Source: CAD feature listing. Evaluate the final solid. Frame: model axes, mm. A direction names the side the tool comes from. Round coordinates to 2 decimals unless told otherwise and drop trailing zeros. Write each loop counter-clockwise with the first axis right and the second up, starting at its lowest first coordinate (ties: lowest second). Pieces come first, ordered by that corner, then holes. Notation, with made-up numbers: (-31, 72.25) - (4, 72.25) arc R5 ccw to (4, 81.25) - close; hole circle Ø3 at (21, 54.25). An arc over 180 degrees is marked (long way). Write item = value, one per line. Start each with the question number.
```python
from build123d import *

# Parameters (mm, degrees)
SKETCH_1_R      = 2.5
SKETCH_1_R_2    = 2.25
EXTRUDE_1_DEPTH = 2.5
FILLET_1_R      = 2


with BuildPart() as part:
    # 草图1 → 拉伸1 (new body)
    with BuildSketch(Plane.XY):
        with BuildLine():
            Line((-3.85, -23), (-3.85, -7.578093428))
            ThreePointArc((-3.85, -7.578093428), (0.055897166, 8.499816204), (3.75, -7.628073151))
            Line((3.75, -7.628073151), (3.75, -23))
            Line((3.75, -23), (-3.85, -23))
        make_face()
        Circle(SKETCH_1_R, mode=Mode.SUBTRACT)
        with Locations((0, -19)):
            Circle(SKETCH_1_R_2, mode=Mode.SUBTRACT)
    extrude(amount=EXTRUDE_1_DEPTH)

    # 圆角1
    fillet_1_edges = [part.edges().sort_by_distance(p)[0] for p in [
        (-3.85, -23, 1.25),
        (-3.85, -7.578093428, 1.25),
        (3.75, -7.628073151, 1.25),
        (3.75, -23, 1.25),
    ]]
    fillet(fillet_1_edges, radius=FILLET_1_R)


solid = part.part
```
(1) Section A-A (y = 0). Return the cut outline in (x, z).
(2) Reachability of faces 1 (the flat face through (-3.85, -15, 1)), 2 (the flat face through (3.75, -15, 1)), 3 (the cylindrical face through (-0.488, -21.196, 1.232)) from +Z, -Z, +X, -X, +Y, -Y: full face, straight path, thin tool, end or side. Return the list, or none.
(3) Section D-D (y = -19). Return the cut outline in (x, z).
(4) Contact query for flat-ended pins moving along their axis: P1, Ø1, axis at y = 1.5, z = 1, coming from the -X side; P2, Ø0.8, axis at y = -15, z = 1.5, coming from the -X side. Output: stop coordinate, or through.
(5) Section C-C (z = 0.3). Return the cut outline in (x, y), plus the area to 3 significant figures.
(6) Section B-B (x = 0). Return the cut outline in (y, z).
(7) Pull-direction query (X, two-part tool) for faces 4 (the cylindrical face through (-0.54, -2.44, 1.23)), 5 (the cylindrical face through (4, -7.82, 1.27)), 6 (the flat face through (0, -4, 0)), 7 (the cylindrical face through (-3.28, -22.4, 1.27)); classes: +X half, -X half, draft (parallel to the pull), parting line (faces both ways), or undercut.
(8) Ray query, L1, parallel to Y at x = 0, z = 0.3; L2, parallel to Y at x = 0.5, z = 2.3; L3, parallel to X at y = -14.5, z = 2.1. Return the intervals inside material, ascending. Write a range as from..to.
Solution:
q1.outline = (-8.5, 0) - (-2.5, 0) - (-2.5, 2.5) - (-8.5, 2.5) - close; (2.5, 0) - (8.5, 0) - (8.5, 2.5) - (2.5, 2.5) - close
q2.face_1 = +Z, -Z, -X, -Y
q2.face_2 = +Z, -Z, +X, -Y
q2.face_3 = +Z, -Z
q3.outline = (-3.85, 0) - (-2.25, 0) - (-2.25, 2.5) - (-3.85, 2.5) - close; (2.25, 0) - (3.75, 0) - (3.75, 2.5) - (2.25, 2.5) - close
q4.P1 = -8.44
q4.P2 = -3.85
q5.outline = (-4.74, -7.06) arc R2 cw to (-3.85, -8.72) - (-3.85, -21) arc R2 ccw to (-1.85, -23) - (1.75, -23) arc R2 ccw to (3.75, -21) - (3.75, -8.79) arc R2 cw to (4.65, -7.11) arc R8.5 ccw (long way) to start; hole circle Ø5 at (0, 0); hole circle Ø4.5 at (0, -19)
q5.area = 303 mm^2
q6.outline = (-23, 0) - (-21.25, 0) - (-21.25, 2.5) - (-23, 2.5) - close; (-16.75, 0) - (-2.5, 0) - (-2.5, 2.5) - (-16.75, 2.5) - close; (2.5, 0) - (8.5, 0) - (8.5, 2.5) - (2.5, 2.5) - close
q7.face_4 = undercut
q7.face_5 = +X half
q7.face_6 = draft
q7.face_7 = -X half
q8.L1 = -23..-21.25, -16.75..-2.5, 2.5..8.5
q8.L2 = -23..-21.19, -16.81..-2.45, 2.45..8.49
q8.L3 = -3.85..3.75
